```python
from build123d import *

# Parameters (mm, degrees)
F0_R     = 18
F0_R_2   = 6
F1_DEPTH = 30


with BuildPart() as f1:
    # F0 (on Front) → F1 (new body, symmetric)
    with BuildSketch(Plane.XZ):
        with BuildLine():
            Line((3.25, -24.78785), (101.56, -11.898168))
            ThreePointArc((101.56, -11.898168), (112, 0), (101.56, 11.898168))
            Line((101.56, 11.898168), (3.25, 24.78785))
            ThreePointArc((3.25, 24.78785), (-25, 0), (3.25, -24.78785))
        make_face()
        Circle(F0_R, mode=Mode.SUBTRACT)
        with BuildLine():
            ThreePointArc((25.077968, 6.862616), (26.13184, 11.468083), (30.550655, 13.13992))
            Line((30.550655, 13.13992), (80.18, 6.632887))
            ThreePointArc((80.18, 6.632887), (86, 0), (80.18, -6.632887))
            Line((80.18, -6.632887), (30.550655, -13.13992))
            ThreePointArc((30.550655, -13.13992), (26.13184, -11.468083), (25.077968, -6.862616))
            ThreePointArc((25.077968, -6.862616), (26, 0), (25.077968, 6.862616))
        make_face(mode=Mode.SUBTRACT)
        with Locations((100, 0)):
            Circle(F0_R_2, mode=Mode.SUBTRACT)
    extrude(amount=F1_DEPTH, both=True)


solid = f1.part
```
For this review, take the finished solid that the model builds, in its own axes (mm). A direction names the side the tool comes from. Round coordinates to 2 decimals unless told otherwise and drop trailing zeros. Loops run counter-clockwise (first coordinate to the right, second up) from the corner with the lowest first, then second, coordinate; pieces in that order, holes last.
(1) We need section B-B (x = 0). Give the boundary of the cut face in (y, z), plus the area to 3 significant figures.
Returned:
outline: (-30, -25) - (30, -25) - (30, -18) - (-30, -18) - close; (-30, 18) - (30, 18) - (30, 25) - (-30, 25) - close
area: 840 mm2
(2) Tool access review of faces 1 (the flat face through (43, 30, -16)), 2 (the cylindrical face through (26, 0, 0)): name each direction out of +Z, -Z, +X, -X, +Y, -Y from which nothing blocks a thin tool from reaching the whole face with its end or side.
Returned:
face 1: +Z, -Z, +X, -X, +Y
face 2: +Y, -Y
(3) We need section D-D (x = 100). Give the boundary of the cut face in (y, z), plus the area to 3 significant figures.
Returned:
outline: (-30, -12.1) - (30, -12.1) - (30, -6) - (-30, -6) - close; (-30, 6) - (30, 6) - (30, 12.1) - (-30, 12.1) - close
area: 732 mm2
(4) We need section A-A (z = 0). Give the boundary of the cut face in (x, y).
Returned:
outline: (-25, -30) - (-18, -30) - (-18, 30) - (-25, 30) - close; (18, -30) - (26, -30) - (26, 30) - (18, 30) - close; (86, -30) - (94, -30) - (94, 30) - (86, 30) - close; (106, -30) - (112, -30) - (112, 30) - (106, 30) - close
(5) We need section C-C (y = -5). Give the boundary of the cut face in (x, z).
Returned:
outline: (3.25, -24.79) - (101.56, -11.9) arc R12 ccw to (101.56, 11.9) - (3.25, 24.79) arc R25 ccw (long way) to start; hole circle Ø36 at (0, 0); hole (25.08, -6.86) arc R5 ccw to (30.55, -13.14) - (80.18, -6.63) arc R6.69 ccw to (80.18, 6.63) - (30.55, 13.14) arc R5 ccw to (25.08, 6.86) arc R26 cw to start; hole circle Ø12 at (100, 0)
(6) Clearance check with flat-ended pins moving along their axes: P1, Ø1.5, axis at x = 82, y = 5.5, coming from the -Z side; P2, Ø3, axis at x = 96.5, y = -3.5, coming from the -Z side; P3, Ø8, axis at x = 3.5, y = -14, coming from the +Z side; P4, Ø1.5, axis at x = 41, y = 4, coming from the -Z side. State where each tip first meets the part, or that it passes through.
Returned:
P1: stops at z = -14.56
P2: stops at z = -12.76
P3: stops at z = 25
P4: stops at z = -19.94
(7) Wall thickness on line 1 along X through (y, z) = (-11, -4); line 2 along Z through (x, y) = (102, -1); line 3 along Z through (x, y) = (59.5, 8): over which ranges is each line inside the solid? List them lowest first.
Returned:
line 1: x = -24.68 to -17.55, 17.55 to 25.69, 84.67 to 95.53, 104.47 to 111.31
line 2: z = -11.83 to -5.66, 5.66 to 11.83
line 3: z = -17.41 to -9.34, 9.34 to 17.41
(8) Mouldability with a two-part tool opening along X and no side actions: class faces 3 (the cylindrical face through (26.18, -0.42, -11.52)), 4 (the flat face through (53.093, -0.42, 18.253)), 5 (the flat face through (43, -30, -16)) as released by +X, released by -X, zero draft, split by the parting line, or undercut.
Returned:
face 3: undercut
face 4: released by +X
face 5: zero draft
